Input: dimensioned drawing with shaded views. Units: mm. Origin: part minimum x, y, z. A direction names the side the tool comes from. Round coordinates to 2 decimals unless told otherwise and drop trailing zeros. Write each loop counter-clockwise with the first axis right and the second up, starting at its lowest first coordinate (ties: lowest second). Pieces come first, ordered by that corner, then holes. Notation, with made-up numbers: M 56.5,-7.75 L 80.5,-7.75 A15 ccw 80.5,-1.75 Z; hole C 25,20.25 d7. An arc over 180 degrees is marked long. Answer in a Markdown table with one row per item. Add a question column.
Item 1: Cut plane D-D on z = 10. Return loops of the section in (x, y).
Item 2: Mould query, pull axis X, two halves, no side actions, for the marked faces 3, 4, 5 and 6. Classes: released by +X, released by -X, zero draft, split by the parting line, or undercut.
Item 3: Contact query for flat-ended pins moving along their axis: pin 1 (1 mm diameter, centred on x = 19, y = 6.5, fed in from +Z); pin 2 (4 mm diameter, centred on x = 15.5, z = 2.5, fed in from -Y); pin 3 (2 mm diameter, centred on x = 8, z = 1.5, fed in from +Y); pin 4 (1.8 mm diameter, centred on x = 16, y = 5, fed in from +Z). Output: stop coordinate, or through.
Item 4: Cut plane B-B on z = 12.5. Return loops of the section in (x, y).
Item 5: Set-up query: the marked faces 1 and 2. Return all of +Z, -Z, +X, -X, +Y, -Y with unobstructed straight access to the full face (end or side cutting, diameter ignored); none if empty.
Item 6: Material intervals for probe 1 along Y at (x, z) = (16, 0.4); probe 2 along X at (y, z) = (17, 11.25); probe 3 along Z at (x, y) = (6, 1.5), sorted ascending.
Item 7: Cut plane C-C on y = 6. Return loops of the section in (x, z).
Item 8: Cut plane A-A on x = 16. Return loops of the section in (y, z).
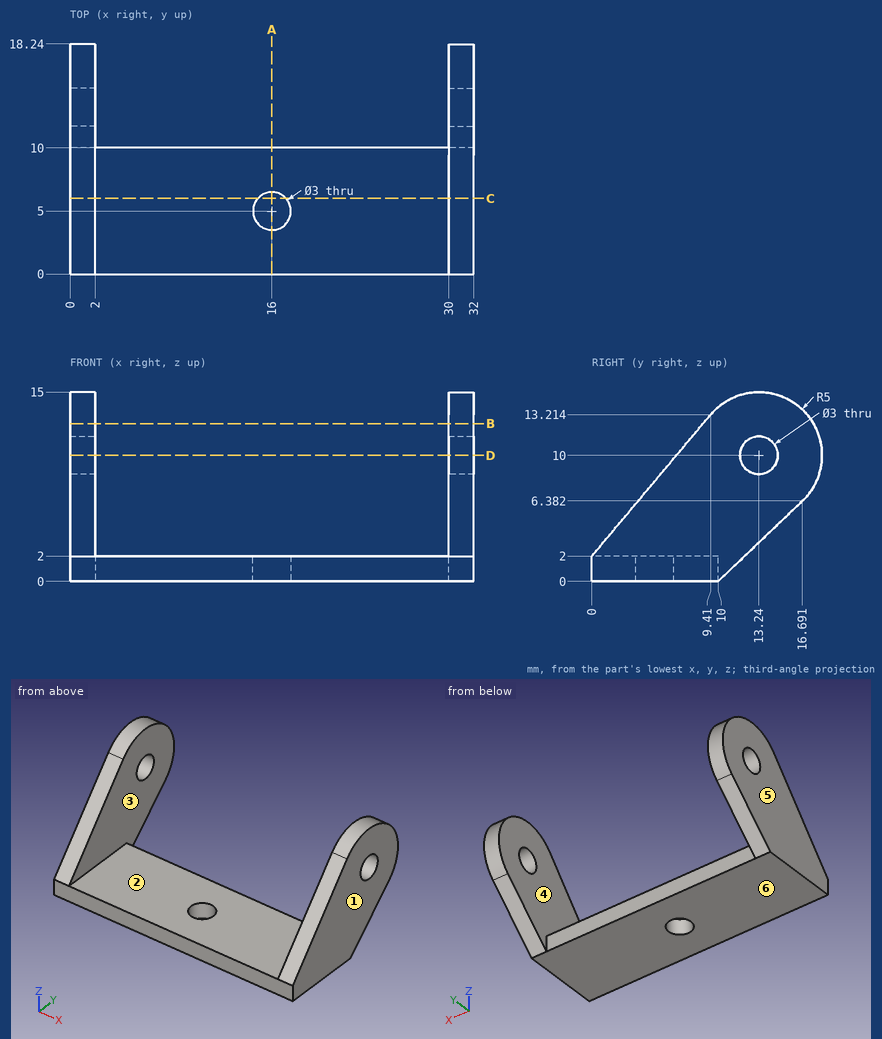
Results below:
| question | item | result |
|---|---|---|
| 1 | outline | M 0,6.71 L 2,6.71 L 2,11.74 L 0,11.74 Z; M 0,14.74 L 2,14.74 L 2,18.24 L 0,18.24 Z; M 30,6.71 L 32,6.71 L 32,11.74 L 30,11.74 Z; M 30,14.74 L 32,14.74 L 32,18.24 L 30,18.24 Z |
| 2 | face 3 | undercut |
| 2 | face 4 | undercut |
| 2 | face 5 | released by -X |
| 2 | face 6 | zero draft |
| 3 | pin 1 | z = 2 |
| 3 | pin 2 | y = 0 |
| 3 | pin 3 | y = 10 |
| 3 | pin 4 | through |
| 4 | outline | M 0,8.81 L 2,8.81 L 2,17.57 L 0,17.57 Z; M 30,8.81 L 32,8.81 L 32,17.57 L 30,17.57 Z |
| 5 | face 1 | +Z, -Z, +X, +Y, -Y |
| 5 | face 2 | +Z, +Y, -Y |
| 6 | probe 1 | 0 to 3.5, 6.5 to 10 |
| 6 | probe 2 | 0 to 2, 30 to 32 |
| 6 | probe 3 | 0 to 2 |
| 7 | outline | M 0,0 L 14.88,0 L 14.88,2 L 2,2 L 2,9.15 L 0,9.15 Z; M 17.12,0 L 32,0 L 32,9.15 L 30,9.15 L 30,2 L 17.12,2 Z |
| 8 | outline | M 0,0 L 3.5,0 L 3.5,2 L 0,2 Z; M 6.5,0 L 10,0 L 10,2 L 6.5,2 Z |
